The model under review builds one solid part; all positions refer to its coordinate system, in mm. Give positions to 0.01 mm unless a question says otherwise; leave off trailing zeros. Write each loop counter-clockwise with the first axis right and the second up, starting at its lowest first coordinate (ties: lowest second). Pieces come first, ordered by that corner, then holes. Notation, with made-up numbers: (-25.75, -8) - (4.25, -8) arc R21 ccw to (4.25, 21) - close; hole circle Ø3 at (63.5, -39.5). An arc over 180 degrees is marked (long way). Write item = value, one per line.
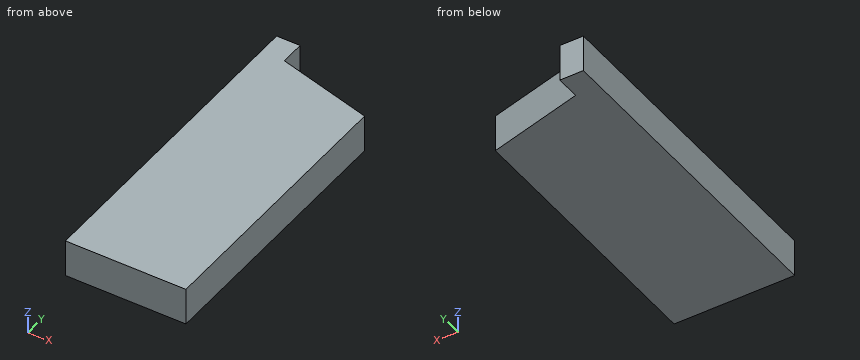
```python
from build123d import *

# Parameters (mm, degrees)
EXTRUDE_1_DEPTH          = 7.6
CUT_EXTRUDE_1_DEPTH      = 72.697539881
CUT_EXTRUDE_1_DEPTH_BACK = 72.697539881


with BuildPart() as part:
    # 草图1 → 凸台-拉伸1 (new body)
    with BuildSketch(Plane.XY):
        Polygon((4.8, 0), (0, 0), (0, -66.915), (24.6, -66.915), (24.6, 0), (19.8, 0), (19.8, -5), (4.8, -5), align=None)
    extrude(amount=EXTRUDE_1_DEPTH)

    # 草图2 → 切除-拉伸1 (cut, two sides: drawn at the far end of the back side and taken through both)
    with BuildSketch(Plane.XY.offset(7.6).offset(-CUT_EXTRUDE_1_DEPTH_BACK)):
        Polygon((19.8, -5), (4.8, -5), (24.6, -10.30539401), (24.6, 0), (19.8, 0), align=None)
    extrude(amount=CUT_EXTRUDE_1_DEPTH + CUT_EXTRUDE_1_DEPTH_BACK, mode=Mode.SUBTRACT)


solid = part.part
```
1. Take a section at C-C on y = -7.5. Give the boundary of the cut face in (x, z), and give its area (3 significant figures).
Findings below:
outline = (0, 0) - (14.13, 0) - (14.13, 7.6) - (0, 7.6) - close
area = 107 mm²
2. Take a section at A-A on z = 6. Give the boundary of the cut face in (x, y) (3 decimals).
Findings below:
outline = (0, -66.915) - (24.6, -66.915) - (24.6, -10.305) - (4.8, -5) - (4.8, 0) - (0, 0) - close
3. For line 1 (Y direction, x = 16.5, z = 2.25) (3 decimals); line 2 (X direction, y = -3, z = 7); line 3 (Y direction, x = 19.25, z = 6.25) (3 decimals), list the stretches that pass through material, from the lowest coordinate up. Write a range as from..to.
Findings below:
line_1 = -66.915..-8.135
line_2 = 0..4.8
line_3 = -66.915..-8.872
4. Insertion check: P1, Ø3, axis at x = 12.5, z = 2, coming from the +Y side; P2, Ø2.5, axis at y = -1.5, z = 5, coming from the +X side. Each pin has a flat end and moves straight along its axis. Give the tip position at first contact, or say it passes through.
Findings below:
P1 = -6.66
P2 = 4.8
5. Take a section at B-B on x = 12.25. Give the boundary of the cut face in (y, z) (3 decimals), and give its area (3 significant figures).
Findings below:
outline = (-66.915, 0) - (-6.996, 0) - (-6.996, 7.6) - (-66.915, 7.6) - close
area = 455 mm²
